Here's how the part is built. I have some questions about the finished solid (model axes, mm). Round coordinates to 2 decimals unless told otherwise and drop trailing zeros. Write each loop counter-clockwise with the first axis right and the second up, starting at its lowest first coordinate (ties: lowest second). Pieces come first, ordered by that corner, then holes. Notation, with made-up numbers: M 53,38 L 95,38 A16 cw 95,59 Z; hole C 69.25,48.5 d5. An arc over 180 degrees is marked long. Use one line per item in the form item = value. Start each with the question number.
Q1. I want a section at C-C on y = 99. List the corners of the cut face in (x, z) for me, and give its area (3 significant figures).
Q2. I want a section at B-B on y = 85. List the corners of the cut face in (x, z) for me, and give its area (3 significant figures).
Q3. I want a section at A-A on x = 75.5. List the corners of the cut face in (y, z) for me.
Q4. I'm going to push flat-ended pins straight in: pin 1 Ø10 at (x, y) = (42.5, 59) entering from -Z; pin 2 Ø0.6 at (x, z) = (67.5, 1) entering from -Y; pin 3 Ø1 at (x, z) = (3, 1) entering from +Y. Where does each tip first touch, or does it pass through?
Q5. I want a section at D-D on z = 1. State how many separate pieces and enclosed holes the cut face has, and give its area (3 significant figures).
Q6. I need wall thicknesses on line 1 along Y through (x, z) = (51, 1.75); line 2 along Y through (x, z) = (118, 1); line 3 along X through (y, z) = (27, 0.8). Which ranges of each line are inside material? Lowest first, please. Write a range as from..to.
```python
from build123d import *

# Parameters (mm, degrees)
PAD_DEPTH                 = 2
PAD_LINEARPATTERN_2_DEPTH = 2
PAD_LINEARPATTERN_3_DEPTH = 2
LINEARPATTERN001_COUNT    = 4
LINEARPATTERN001_PITCH    = 26.666667


with BuildPart() as part:
    # Sketch → Pad (new body)
    with BuildSketch(Plane.XY):
        Polygon((7.488891, 13.894065), (-7.934416, 13.894065), (-16, 0), (-8, -13.856406), (8, -13.856406), (16, 0), (31.852406, 0), (39.484819, 13.894065), (31.413057, 27.537577), (15.560652, 27.537577), align=None)
        Polygon((-15, 0), (-7.5, -12.990381), (7.5, -12.990381), (15, 0), (7.5, 12.990381), (-7.5, 12.990381), align=None, mode=Mode.SUBTRACT)
        Polygon((8.486855, 13.638825), (15.986855, 0.648444), (30.986855, 0.648444), (38.486855, 13.638825), (30.986855, 26.629206), (15.986855, 26.629206), align=None, mode=Mode.SUBTRACT)
    pad = extrude(amount=PAD_DEPTH)

    # Sketch LinearPattern 2 → Pad LinearPattern 2 (add)
    with BuildSketch(Plane(origin=(47, 0, 0), x_dir=(1, 0, 0), z_dir=(0, 0, 1))):
        Polygon((7.488891, 13.894065), (-7.934416, 13.894065), (-16, 0), (-8, -13.856406), (8, -13.856406), (16, 0), (31.852406, 0), (39.484819, 13.894065), (31.413057, 27.537577), (15.560652, 27.537577), align=None)
        Polygon((-15, 0), (-7.5, -12.990381), (7.5, -12.990381), (15, 0), (7.5, 12.990381), (-7.5, 12.990381), align=None, mode=Mode.SUBTRACT)
        Polygon((8.486855, 13.638825), (15.986855, 0.648444), (30.986855, 0.648444), (38.486855, 13.638825), (30.986855, 26.629206), (15.986855, 26.629206), align=None, mode=Mode.SUBTRACT)
    pad_linearpattern_2 = extrude(amount=PAD_LINEARPATTERN_2_DEPTH)

    # Sketch LinearPattern 3 → Pad LinearPattern 3 (add)
    with BuildSketch(Plane(origin=(94, 0, 0), x_dir=(1, 0, 0), z_dir=(0, 0, 1))):
        Polygon((7.488891, 13.894065), (-7.934416, 13.894065), (-16, 0), (-8, -13.856406), (8, -13.856406), (16, 0), (31.852406, 0), (39.484819, 13.894065), (31.413057, 27.537577), (15.560652, 27.537577), align=None)
        Polygon((-15, 0), (-7.5, -12.990381), (7.5, -12.990381), (15, 0), (7.5, 12.990381), (-7.5, 12.990381), align=None, mode=Mode.SUBTRACT)
        Polygon((8.486855, 13.638825), (15.986855, 0.648444), (30.986855, 0.648444), (38.486855, 13.638825), (30.986855, 26.629206), (15.986855, 26.629206), align=None, mode=Mode.SUBTRACT)
    pad_linearpattern_3 = extrude(amount=PAD_LINEARPATTERN_3_DEPTH)

    # LinearPattern001: Pad, Pad LinearPattern 2, Pad LinearPattern 3 ×4
    with Locations(*[(0, i * LINEARPATTERN001_PITCH, 0) for i in range(1, LINEARPATTERN001_COUNT)]):
        add(pad)
        add(pad_linearpattern_2)
        add(pad_linearpattern_3)


solid = part.part
```
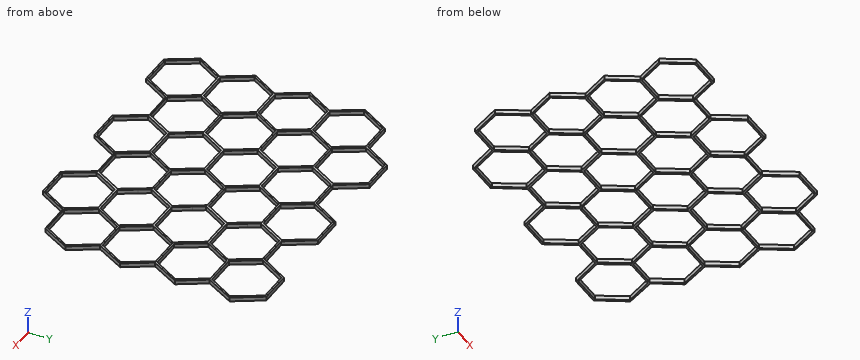
Reported:
q1.outline = M 10.51,0 L 11.58,0 L 11.58,2 L 10.51,2 Z; M 35.39,0 L 36.46,0 L 36.46,2 L 35.39,2 Z; M 57.51,0 L 58.58,0 L 58.58,2 L 57.51,2 Z; M 82.39,0 L 83.46,0 L 83.46,2 L 82.39,2 Z; M 104.51,0 L 105.58,0 L 105.58,2 L 104.51,2 Z; M 129.39,0 L 130.46,0 L 130.46,2 L 129.39,2 Z
q1.area = 12.9 mm^2
q2.outline = M -13.1,0 L -12.11,0 L -12.11,2 L -13.1,2 Z; M 12.11,0 L 13.47,0 L 13.47,2 L 12.11,2 Z; M 33.5,0 L 34.89,0 L 34.89,2 L 33.5,2 Z; M 59.11,0 L 60.47,0 L 60.47,2 L 59.11,2 Z; M 80.5,0 L 81.89,0 L 81.89,2 L 80.5,2 Z; M 106.11,0 L 107.47,0 L 107.47,2 L 106.11,2 Z; M 127.5,0 L 128.6,0 L 128.6,2 L 127.5,2 Z
q2.area = 17.9 mm^2
q3.outline = M 0,0 L 0.65,0 L 0.65,2 L 0,2 Z; M 26.63,0 L 27.54,0 L 27.54,2 L 26.63,2 Z; M 53.3,0 L 54.2,0 L 54.2,2 L 53.3,2 Z; M 79.96,0 L 80.87,0 L 80.87,2 L 79.96,2 Z; M 106.63,0 L 107.54,0 L 107.54,2 L 106.63,2 Z
q4.pin_1 = through
q4.pin_2 = 0
q4.pin_3 = 93.89
q5.separate_pieces = 1
q5.enclosed_holes = 24
q5.area = 1,350 mm^2
q6.line_1 = -13.86..-12.99, 12.81..13.89, 39.48..40.56, 66.14..67.23, 92.99..93.89
q6.line_2 = 0..0.65, 26.63..27.54, 53.3..54.2, 79.96..80.87, 106.63..107.54
q6.line_3 = -15.81..-14.81, 14.81..32.19, 61.81..79.19, 108.81..126.04
